Geometry: final body of the model. Coordinates: model frame, mm. Round coordinates to 2 decimals unless told otherwise and drop trailing zeros. Loops run counter-clockwise (first coordinate to the right, second up) from the corner with the lowest first, then second, coordinate; pieces in that order, holes last. Notation, with made-up numbers: M 37.25,55 L 51.25,55 A27 ccw 51.25,71 Z; hole C 78,4 d1. An arc over 180 degrees is marked long. Return JSON: item names as keys, results as strings.
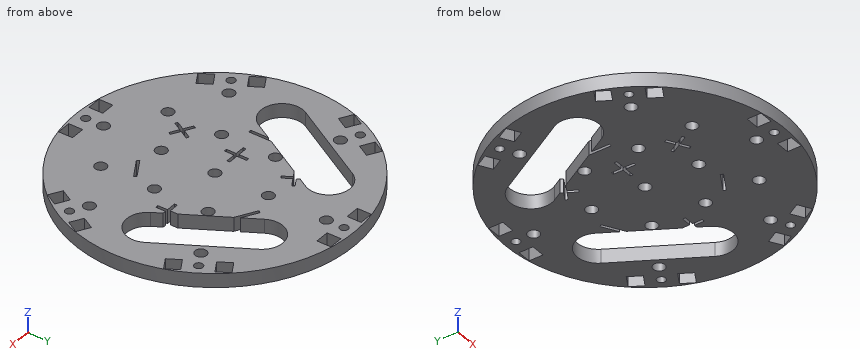
from build123d import *

# Parameters (mm, degrees)
BOSS_EXTRU_1_OUTLINE_R   = 50
BOSS_EXTRU_1_OUTLINE_W   = 5
BOSS_EXTRU_1_OUTLINE_H   = 5
BOSS_EXTRU_1_OUTLINE_R_2 = 2.05
BOSS_EXTRU_1_OUTLINE_R_3 = 1.5
BOSS_EXTRU_1_DEPTH       = 5
SKETCH3_W                = 1
SKETCH3_H                = 8
CUT_EXTRUDE2_DEPTH       = 10
CUT_EXTRUDE3_DEPTH       = 10


# Read off the part's stored shape, not the designer's step: Boss.-Extru.1
with BuildPart() as part:
    # Boss.-Extru.1 outline → Boss.-Extru.1 (new body)
    with BuildSketch(Plane.XY):
        Circle(BOSS_EXTRU_1_OUTLINE_R)
        Polygon((-37.262039705, -33.060254038), (-39.762039705, -28.730127019), (-35.431912686, -26.230127019), (-32.931912686, -30.560254038), align=None, mode=Mode.SUBTRACT)
        with Locations((-7.5, -46.3)):
            Rectangle(BOSS_EXTRU_1_OUTLINE_W, BOSS_EXTRU_1_OUTLINE_H, mode=Mode.SUBTRACT)
        with Locations((-16.666666667, -28.867513459)):
            Circle(BOSS_EXTRU_1_OUTLINE_R_2, mode=Mode.SUBTRACT)
        with Locations((-40.096976195, -23.15)):
            Circle(BOSS_EXTRU_1_OUTLINE_R_3, mode=Mode.SUBTRACT)
        Polygon((-42.931912686, -13.239745962), (-40.431912686, -17.569872981), (-44.762039705, -20.069872981), (-47.262039705, -15.739745962), align=None, mode=Mode.SUBTRACT)
        with Locations((-34.597845014, -19.975075132)):
            Circle(BOSS_EXTRU_1_OUTLINE_R_2, mode=Mode.SUBTRACT)
        with Locations((-16.671397033, -9.625235564)):
            Circle(BOSS_EXTRU_1_OUTLINE_R_2, mode=Mode.SUBTRACT)
        with Locations((0, -46.3)):
            Circle(BOSS_EXTRU_1_OUTLINE_R_3, mode=Mode.SUBTRACT)
        with Locations((7.5, -46.3)):
            Rectangle(BOSS_EXTRU_1_OUTLINE_W, BOSS_EXTRU_1_OUTLINE_H, mode=Mode.SUBTRACT)
        with Locations((0, -39.950150265)):
            Circle(BOSS_EXTRU_1_OUTLINE_R_2, mode=Mode.SUBTRACT)
        with Locations((16.666666667, -28.867513459)):
            Circle(BOSS_EXTRU_1_OUTLINE_R_2, mode=Mode.SUBTRACT)
        Polygon((32.931912686, -30.560254038), (35.431912686, -26.230127019), (39.762039705, -28.730127019), (37.262039705, -33.060254038), align=None, mode=Mode.SUBTRACT)
        with Locations((0, -19.232757636)):
            Circle(BOSS_EXTRU_1_OUTLINE_R_2, mode=Mode.SUBTRACT)
        with Locations((16.666666667, -9.622504487)):
            Circle(BOSS_EXTRU_1_OUTLINE_R_2, mode=Mode.SUBTRACT)
        with Locations((34.597845014, -19.975075132)):
            Circle(BOSS_EXTRU_1_OUTLINE_R_2, mode=Mode.SUBTRACT)
        with Locations((40.096976195, -23.15)):
            Circle(BOSS_EXTRU_1_OUTLINE_R_3, mode=Mode.SUBTRACT)
        Polygon((47.262039705, -15.739745962), (44.762039705, -20.069872981), (40.431912686, -17.569872981), (42.931912686, -13.239745962), align=None, mode=Mode.SUBTRACT)
        with Locations((-33.333333333, 0)):
            Circle(BOSS_EXTRU_1_OUTLINE_R_2, mode=Mode.SUBTRACT)
        Polygon((-47.262039705, 15.739745962), (-44.762039705, 20.069872981), (-40.431912686, 17.569872981), (-42.931912686, 13.239745962), align=None, mode=Mode.SUBTRACT)
        with Locations((-40.096976195, 23.15)):
            Circle(BOSS_EXTRU_1_OUTLINE_R_3, mode=Mode.SUBTRACT)
        with Locations((-34.597845014, 19.975075132)):
            Circle(BOSS_EXTRU_1_OUTLINE_R_2, mode=Mode.SUBTRACT)
        with Locations((-16.671397032, 9.625235564)):
            Circle(BOSS_EXTRU_1_OUTLINE_R_2, mode=Mode.SUBTRACT)
        Polygon((-32.931912686, 30.560254038), (-35.431912686, 26.230127019), (-39.762039705, 28.730127019), (-37.262039705, 33.060254038), align=None, mode=Mode.SUBTRACT)
        with Locations((-16.666666667, 28.867513459)):
            Circle(BOSS_EXTRU_1_OUTLINE_R_2, mode=Mode.SUBTRACT)
        with Locations((-7.5, 46.3)):
            Rectangle(BOSS_EXTRU_1_OUTLINE_W, BOSS_EXTRU_1_OUTLINE_H, mode=Mode.SUBTRACT)
        Circle(BOSS_EXTRU_1_OUTLINE_R_2, mode=Mode.SUBTRACT)
        with Locations((16.669571796, 9.624181764)):
            Circle(BOSS_EXTRU_1_OUTLINE_R_2, mode=Mode.SUBTRACT)
        with Locations((0, 19.165334425)):
            Circle(BOSS_EXTRU_1_OUTLINE_R_2, mode=Mode.SUBTRACT)
        with Locations((33.333333333, 0)):
            Circle(BOSS_EXTRU_1_OUTLINE_R_2, mode=Mode.SUBTRACT)
        with Locations((34.597845014, 19.975075133)):
            Circle(BOSS_EXTRU_1_OUTLINE_R_2, mode=Mode.SUBTRACT)
        Polygon((42.931912686, 13.239745962), (40.431912686, 17.569872981), (44.762039705, 20.069872981), (47.262039705, 15.739745962), align=None, mode=Mode.SUBTRACT)
        with Locations((40.096976195, 23.15)):
            Circle(BOSS_EXTRU_1_OUTLINE_R_3, mode=Mode.SUBTRACT)
        with Locations((16.666666667, 28.867513459)):
            Circle(BOSS_EXTRU_1_OUTLINE_R_2, mode=Mode.SUBTRACT)
        with Locations((0, 39.950150265)):
            Circle(BOSS_EXTRU_1_OUTLINE_R_2, mode=Mode.SUBTRACT)
        with Locations((0, 46.3)):
            Circle(BOSS_EXTRU_1_OUTLINE_R_3, mode=Mode.SUBTRACT)
        with Locations((7.5, 46.3)):
            Rectangle(BOSS_EXTRU_1_OUTLINE_W, BOSS_EXTRU_1_OUTLINE_H, mode=Mode.SUBTRACT)
        Polygon((37.262039705, 33.060254038), (39.762039705, 28.730127019), (35.431912686, 26.230127019), (32.931912686, 30.560254038), align=None, mode=Mode.SUBTRACT)
    extrude(amount=BOSS_EXTRU_1_DEPTH)

    # Sketch3 → Cut-Extrude2 (cut)
    with BuildSketch(Plane.XY.offset(5)):
        with Locations((-22.833333333, 0)):
            Rectangle(SKETCH3_W, SKETCH3_H)
        Polygon((-13.233653965, 23.921361037), (-14.099679369, 23.421361037), (-12.349679369, 20.390272124), (-15.380768282, 18.640272124), (-14.880768282, 17.77424672), (-11.849679369, 19.52424672), (-10.099679369, 16.493157806), (-9.233653965, 16.993157806), (-10.983653965, 20.02424672), (-7.952565052, 21.77424672), (-8.452565052, 22.640272124), (-11.483653965, 20.890272124), align=None)
        Polygon((15.130768282, 18.207259422), (14.630768282, 17.341234018), (7.702565052, 21.341234018), (8.202565052, 22.207259422), align=None)
        Polygon((8.202565052, -22.207259422), (7.702565052, -21.341234018), (14.630768282, -17.341234018), (15.130768282, -18.207259422), align=None)
        Polygon((27.333333333, -0.5), (27.333333333, 0.5), (23.833333333, 0.5), (23.833333333, 4), (22.833333333, 4), (22.833333333, 0.5), (19.333333333, 0.5), (19.333333333, -0.5), (22.833333333, -0.5), (22.833333333, -4), (23.833333333, -4), (23.833333333, -0.5), align=None)
        Polygon((-14.099679369, -23.421361037), (-13.233653965, -23.921361037), (-11.483653965, -20.890272124), (-8.452565052, -22.640272124), (-7.952565052, -21.77424672), (-10.983653965, -20.02424672), (-9.233653965, -16.993157806), (-10.099679369, -16.493157806), (-11.849679369, -19.52424672), (-14.880768282, -17.77424672), (-15.380768282, -18.640272124), (-12.349679369, -20.390272124), align=None)
        Polygon((-7.005935602, -0.708643072), (-7.005935602, 0.291356928), (-10.505935602, 0.291356928), (-10.505935602, 3.791356928), (-11.505935602, 3.791356928), (-11.505935602, 0.291356928), (-15.005935602, 0.291356928), (-15.005935602, -0.708643072), (-11.505935602, -0.708643072), (-11.505935602, -4.208643072), (-10.505935602, -4.208643072), (-10.505935602, -0.708643072), align=None)
        Polygon((-20.645633013, 13.413868493), (-21.300480769, 12.280855673), (-21.552183494, 12.425987884), (-20.897335737, 13.559000705), align=None)
    extrude(amount=-CUT_EXTRUDE2_DEPTH, mode=Mode.SUBTRACT)

    # Sketch4 → Cut-Extrude3 (cut)
    with BuildSketch(Plane(origin=(0, 0, 0), x_dir=(-1, 0, 0), z_dir=(0, 0, -1))):
        with BuildLine():
            Line((26.838142805, -3.75), (10.171476138, 25.117513459))
            ThreePointArc((10.171476138, 25.117513459), (12.916666667, 35.362703988), (23.161857195, 32.617513459))
            Line((23.161857195, 32.617513459), (39.828523862, 3.75))
            ThreePointArc((39.828523862, 3.75), (37.083333333, -6.495190528), (26.838142805, -3.75))
        make_face()
        with BuildLine():
            Line((-10.171476138, 25.117513459), (-26.838142805, -3.75))
            ThreePointArc((-26.838142805, -3.75), (-37.083333333, -6.495190528), (-39.828523862, 3.75))
            Line((-39.828523862, 3.75), (-23.161857195, 32.617513459))
            ThreePointArc((-23.161857195, 32.617513459), (-12.916666667, 35.362703988), (-10.171476138, 25.117513459))
        make_face()
    extrude(amount=-CUT_EXTRUDE3_DEPTH, mode=Mode.SUBTRACT)


with BuildPart() as body_2:
    # of the pieces the cut leaves, the one that is kept (cut_extrude3_keep)
    add(part.part.solids().sort_by_distance((50, 0, 0))[0])


solid = body_2.part
Q1. Section query B-B (x = 0). State how many separate pieces and enclosed holes the cut face has, plus the area to 4 significant figures.
Determined:
{"separate pieces": "8", "enclosed holes": "0", "area": "367.5 mm^2"}
Q2. Material intervals for L1, parallel to Y at x = -18, z = 4.5; L2, parallel to X at y = 34, z = 0.5; L3, parallel to X at y = 12.5, z = 2.45, sorted ascending.
Determined:
{"L1": "y = -46.65 to -30.42, -27.31 to -11.19, -8.06 to 8.06, 11.19 to 11.56, 36.25 to 46.65", "L2": "x = -36.66 to -22.14, -11.2 to 11.2, 22.14 to 36.66", "L3": "x = -48.41 to -34.78, -17.46 to 17.46, 34.78 to 48.41"}
Q3. Section query C-C (x = -29.5). Output: boundary loops of the cut face in (y, z), plus the area to 3 significant figures.
Determined:
{"outline": "M -40.37,0 L -6.45,0 L -6.45,5 L -40.37,5 Z; M 21.64,0 L 40.37,0 L 40.37,5 L 21.64,5 Z", "area": "263 mm^2"}
Q4. Section query A-A (y = -46.3). Output: boundary loops of the cut face in (x, z).
Determined:
{"outline": "M -18.88,0 L -10,0 L -10,5 L -18.88,5 Z; M -5,0 L -1.5,0 L -1.5,5 L -5,5 Z; M 1.5,0 L 5,0 L 5,5 L 1.5,5 Z; M 10,0 L 18.88,0 L 18.88,5 L 10,5 Z"}
Q5. Pin query (flat end, axial travel): pin 1 (2 mm diameter, centred on y = -8, z = 2.5, fed in from -X); pin 2 (0.8 mm diameter, centred on x = -11, z = 2.5, fed in from +Y); pin 3 (1.5 mm diameter, centred on y = 46.5, z = 3, fed in from -X). Return the tip coordinate at first contact, or that it passes through.
Determined:
{"pin 1": "stops at x = -49.51", "pin 2": "stops at y = 48.86", "pin 3": "stops at x = -20.17"}
